from build123d import *

# Parameters (mm, degrees)
F4_DEPTH = 0.2
F5_COUNT = 4
F8_DEPTH = 6.0416666667
F9_SIZE  = 0.1


with BuildPart() as f2:
    # F1 (on Front) → F2 (revolve)
    with BuildSketch(Plane.XZ):
        Polygon((0.7986111111, 13.6805555556), (0.7986111111, 0.2604166667), (0.9027777778, 0.5208333333), (0.9027777778, 12.7777777778), align=None)
        with BuildLine():
            Line((0, 31.25), (0, 0))
            Line((0, 0), (0.6944444444, 0))
            Line((0.6944444444, 0), (0.7986111111, 0.2604166667))
            Line((0.7986111111, 0.2604166667), (0.7986111111, 13.6805555556))
            Line((0.7986111111, 13.6805555556), (0.7986111111, 28.9930555556))
            ThreePointArc((0.7986111111, 28.9930555556), (0.7567775283, 29.8651154933), (0.6316609682, 30.7291666667))
            ThreePointArc((0.6316609682, 30.7291666667), (0.4093479388, 31.1030002792), (0, 31.25))
        make_face()
    revolve(axis=Axis((0, 0, 15.625), (0, 0, 1)))

    # F3 (on Front) → F4 (join, symmetric)
    with BuildSketch(Plane.XZ):
        Polygon((0, 27.1527777778), (0, 0.625), (2.7777777778, 0.625), (2.7777777778, 3.75), (1.7361111111, 7.2916666667), (0.4, 8.7391203704), (0.4, 18.9610719875), (3.3680555556, 18.125), (3.0208333333, 20.9027777778), (0.4, 20.3012750455), (0.4, 22.5527777778), (1.5972222222, 23.75), (1.5972222222, 25.5555555556), align=None)
    extrude(amount=F4_DEPTH, both=True)

    # F5: F2 ×4 about axis
    f5_axis = Axis((0, 0, 13.6805555556), (0, 0, 1))


with BuildPart() as f2_1:
    add(f2.part)
    for i in range(1, F5_COUNT):
        add(f2.part.rotate(f5_axis, i * 360 / F5_COUNT))

    # F7 (on offset) → F8 (join)
    with BuildSketch(Plane.XY.offset(18.75)):
        with BuildLine():
            Line((-0.4822828892, -0.777240922), (-0.0760130179, -0.3709710507))
            Line((-0.0760130179, -0.3709710507), (-0.3709710507, -0.0760130179))
            Line((-0.3709710507, -0.0760130179), (-0.777240922, -0.4822828892))
            ThreePointArc((-0.777240922, -0.4822828892), (-0.7090709667, -0.7090709667), (-0.4822828892, -0.777240922))
        make_face()
    extrude(amount=F8_DEPTH)

    # F9
    f9_edges = [f2_1.edges().sort_by_distance(p)[0] for p in [
        (-0.564703, -0.564703, 24.791667),
        (-0.564703, -0.564703, 18.75),
    ]]
    chamfer(f9_edges, length=F9_SIZE)


solid = f2_1.part
For this review, take the finished solid that the model builds, in its own axes (mm). A direction names the side the tool comes from. Give positions to 0.01 mm unless a question says otherwise; leave off trailing zeros. Loops run counter-clockwise (first coordinate to the right, second up) from the corner with the lowest first, then second, coordinate; pieces in that order, holes last. Notation, with made-up numbers: (79, 58) - (108, 58) arc R25 ccw to (108, 78) - close; hole circle Ø1 at (-19, -2.75). An arc over 180 degrees is marked (long way). Write each question's results on one line, items separated by ' | '.
(1) Take a section at D-D (z = 12). Give the boundary of the cut face in (x, y).
Conclusion:
outline: circle Ø1.81 at (0, 0)
(2) Take a section at B-B (y = -2.25). Give the boundary of the cut face in (x, z) (3 decimals), then the cut area to 3 significant figures.
Conclusion:
outline: (-0.2, 0.625) - (0.2, 0.625) - (0.2, 5.544) - (-0.2, 5.544) - close; (-0.2, 18.44) - (0.2, 18.44) - (0.2, 20.726) - (-0.2, 20.726) - close | area: 2.88 mm^2
(3) For line 1 along Z through (x, y) = (0, 1) (3 decimals); line 2 along Y through (x, z) = (-1, 19.5), list the stretches that pass through material, from the lowest coordinate up.
Conclusion:
line 1: 0.625 to 8.089, 18.792 to 20.439, 23.153 to 26.153 | line 2: -0.2 to 0.2
(4) Draft analysis for pull direction Z (two halves, no side actions). For faces 1 (the flat face through (0.2, 1, 25)), 2 (the flat face through (1.19, 0, 25.96)), 3 (the flat face through (1.314, -0.003, 7.749)), state which applies: +Z half, -Z half, draft (parallel to the pull), parting line (faces both ways), or undercut.
Conclusion:
face 1: draft | face 2: +Z half | face 3: undercut
(5) For faces 4 (the flat face through (-0.2, 1, 25)), 5 (the flat face through (1, -0.2, 25)), 6 (the flat face through (-0.2, 2, 4)), 7 (the flat face through (1, 0.2, 25)), list the 3-axis set-ups (+Z, -Z, +X, -X, +Y, -Y) from which the entire face can be reached by the end or side of a thin tool; tool diameter is ignored.
Conclusion:
face 4: +Z, -X, +Y | face 5: +Z, +X, -Y | face 6: +Z, -Z, -X, +Y | face 7: +Z, +X, +Y
(6) Take a section at C-C (z = 6.5). Give the boundary of the cut face in (x, y).
Conclusion:
outline: (-1.97, -0.2) - (-0.88, -0.2) arc R0.9 ccw to (-0.2, -0.88) - (-0.2, -1.97) - (0.2, -1.97) - (0.2, -0.88) arc R0.9 ccw to (0.88, -0.2) - (1.97, -0.2) - (1.97, 0.2) - (0.88, 0.2) arc R0.9 ccw to (0.2, 0.88) - (0.2, 1.97) - (-0.2, 1.97) - (-0.2, 0.88) arc R0.9 ccw to (-0.88, 0.2) - (-1.97, 0.2) - close
(7) For pin 1 Ø1.5 at (x, y) = (2, 0.5) entering from -Z (3 decimals); pin 2 Ø3 at (x, z) = (-2.5, 19) entering from +Y; pin 3 Ø2 at (x, z) = (-1.5, 3.5) entering from -Y, all flat-tipped, find the tip position at first contact; note any pin that passes through.
Conclusion:
pin 1: z = 0.625 | pin 2: y = 0.2 | pin 3: y = -0.75
(8) Take a section at A-A (x = -2). Give the boundary of the cut face in (y, z) (3 decimals), then the cut area to 3 significant figures.
Conclusion:
outline: (-0.2, 0.625) - (0.2, 0.625) - (0.2, 6.394) - (-0.2, 6.394) - close; (-0.2, 18.51) - (0.2, 18.51) - (0.2, 20.668) - (-0.2, 20.668) - close | area: 3.17 mm^2
